Part model, mm, in its own coordinate system. Round coordinates to 2 decimals unless told otherwise and drop trailing zeros. Write each loop counter-clockwise with the first axis right and the second up, starting at its lowest first coordinate (ties: lowest second). Pieces come first, ordered by that corner, then holes. Notation, with made-up numbers: (-8, -33) -> (27, -33) arc R19 cw to (27, -9) -> close; hole circle Ø6 at (86, -10). An arc over 180 degrees is marked (long way). Return JSON: item names as keys, results as strings. Group by question number.
(1) Saw through at B-B (y = 0). State how many separate pieces and enclosed holes the cut face has, plus the area to 3 significant figures.
(2) Saw through at A-A (x = 16). List the corners of the cut face in (y, z).
(3) Drill centre lines: L1, parallel to Y at x = 136, z = 1.5; L2, parallel to Y at x = 72.5, z = 1.9; L3, parallel to Y at x = 82.5, z = 1.95. Where is each one in solid material? Low to high. Write a range as from..to.
from build123d import *

# Parameters (mm, degrees)
ESQUISSE1_R                = 2
BOSS_EXTRU_1_DEPTH         = 2.2
R_P_TITION_LIN_AIRE1_COUNT = 20
R_P_TITION_LIN_AIRE1_PITCH = 8


with BuildPart() as part:
    # Esquisse1 → Boss.-Extru.1 (new body)
    with BuildSketch(Plane.XY):
        Polygon((-1.656854249, -4), (1.656854249, -4), (4, -1.656854249), (4, 1.656854249), (1.656854249, 4), (-1.656854249, 4), (-4, 1.656854249), (-4, -1.656854249), align=None)
        Circle(ESQUISSE1_R, mode=Mode.SUBTRACT)
    boss_extru_1 = extrude(amount=BOSS_EXTRU_1_DEPTH)

    # Répétition linéaire1: Boss.-Extru.1 ×20
    with Locations(*[(i * R_P_TITION_LIN_AIRE1_PITCH, 0, 0) for i in range(1, R_P_TITION_LIN_AIRE1_COUNT)]):
        add(boss_extru_1)


solid = part.part
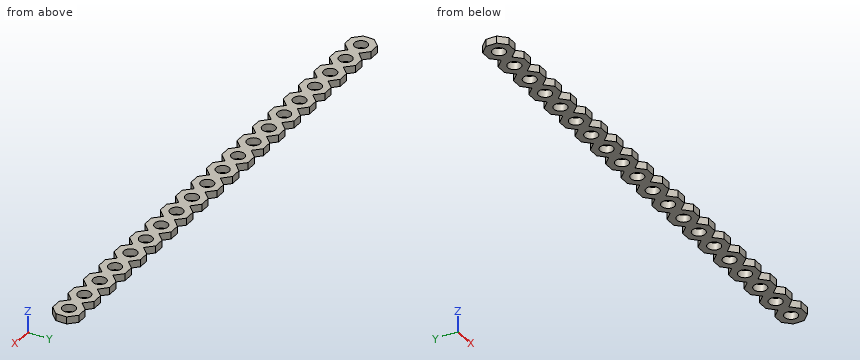
Computed values:
{
 "1": {"separate pieces": "21", "enclosed holes": "0", "area": "176 mm2"},
 "2": {"outline": "(-4, 0) -> (-2, 0) -> (-2, 2.2) -> (-4, 2.2) -> close; (2, 0) -> (4, 0) -> (4, 2.2) -> (2, 2.2) -> close"},
 "3": {"L1": "-4..-2, 2..4", "L2": "-4..-1.94, 1.94..4", "L3": "-3.16..3.16"}
}
